Source: CAD feature listing. Evaluate the final solid. Frame: model axes, mm. Face numbers are marked on the shaded views. A direction names the side the tool comes from. Round coordinates to 2 decimals unless told otherwise and drop trailing zeros. Order: outer loops, then holes, each group sorted by start corner. A loop starts at its lowest first (then second) coordinate and runs counter-clockwise, first axis right, second up. Notation, with made-up numbers: (52.5, 23.5) -> (59.5, 23.5) arc R25 cw to (59.5, 43.5) -> close; hole circle Ø7 at (22, -27). An arc over 180 degrees is marked (long way). Use a Markdown table: item, result. Add a question column.
Autodesk Inventor part; units mm, degrees
ref_plane "Arbeitsebene1" through (-25, 25, -22.5) normal (0, 0, 1) x (1, 0, 0)
ref_plane "YZ Plane" through (0, 0, 0) normal (1, 0, 0) x (0, 1, 0)
ref_plane "XZ Plane" through (0, 0, 0) normal (0, 1, 0) x (-1, 0, 0)
sketch "Skizze1" plane through (0, 0, 0) normal (0, 0, 1) x (1, 0, 0)
  line L0 (-25, 25) -> (25, 25)
  line L1 (25, 25) -> (25, -25)
  line L2 (25, -25) -> (-25, -25)
  line L3 (-25, -25) -> (-25, 25)
  line L4 (-35, 0) -> (35, 0)
  line L5 (0, -35) -> (0, 35)
  line L6 (21, 21) -> (-21, 21)
  line L7 (-21, 21) -> (-21, -21)
  line L8 (-21, -21) -> (21, -21)
  line L9 (21, -21) -> (21, 21)
  point P0 (0, 0)
  dimension "d0" = 50
  dimension "d1" = 50
  dimension "d2" = 4
extrude "Extrusion1" add sketch "Skizze1" along normal blind 45 contours L0 L5 L6 L7 L4 L3 | L0 L1 L4 L9 L6 L5 | L4 L7 L8 L5 L2 L3 | L1 L2 L5 L8 L9 L4
sketch "Skizze2" plane through (-25, -25, 0) normal (-1, 0, 0) x (0, 0, 1)
  line L0 (0, 50) -> (45, 50)
  line L1 (0, 0) -> (45, 0)
  line L2 (22.5, 50) -> (22.5, 0)
  line L3 (0, 46) -> (45, 46)
  line L4 (0, 4) -> (45, 4)
  line L5 (0, 46) -> (5, 46)
  line L6 (10, 41) -> (10, 9)
  line L7 (5, 4) -> (0, 4)
  line L8 (0, 4) -> (0, 46)
  line L9 (45, 4) -> (40, 4)
  line L10 (35, 9) -> (35, 41)
  line L11 (40, 46) -> (45, 46)
  line L12 (45, 46) -> (45, 4)
  arc A0 (40, 46) -> (35, 41) centre (40, 41) ccw
  arc A1 (35, 9) -> (40, 4) centre (40, 9) ccw
  arc A2 (5, 4) -> (10, 9) centre (5, 9) ccw
  arc A3 (10, 41) -> (5, 46) centre (5, 41) ccw
  point P0 (0, 25)
  point P1 (10, 4)
  point P2 (35, 46)
  dimension "d5" = 25
  dimension "d6" = 5
extrude "Extrusion2" cut sketch "Skizze2" against normal up to surface (46 mm away) contours A3 L6 A2 L4 L8 L3 | L3 L12 L4 A1 L10 A0
sketch "Skizze4" plane through (-25, -25, 0) normal (0, -1, 0) x (1, 0, 0)
  line L0 (50, 45) -> (0, 45)
  line L1 (0, 0) -> (0, 45)
  line L2 (50, 0) -> (50, 45)
  line L3 (0, 22.5) -> (50, 22.5)
  line L4 (25, 45) -> (25, 0)
  circle A0 centre (25, 22.5) radius 11
  dimension "d19" = 22
extrude "Extrusion3" cut sketch "Skizze4" against normal up to surface (46 mm away) contours A0 L3 L4 | L4 L3 A0 | A0 L4 L3 | L4 A0 L3
mirror "Spiegeln1" about plane through (0, 0, 0) normal (0, 0, 1) of "Extrusion1", "Extrusion2", "Extrusion3"
sketch "Skizze5" plane through (-25, 25, 45) normal (0, 1, 0) x (1, 0, 0)
  circle A0 centre (33.6603, 27.5) radius 3.45
  circle A1 centre (16.3397, 27.5) radius 3.45
  circle A2 centre (25, 12.5) radius 3.45
  line L0 (0, 0) -> (50, 0)
  line L1 (50, 0) -> (50, 90)
  line L2 (60, 45) -> (-10, 45)
  line L3 (50, 45) -> (0, 45)
  line L4 (0, 45) -> (0, 0)
  line L5 (0, 0) -> (50, 0)
  line L6 (50, 0) -> (50, 45)
  point P0 (25, 45)
extrude "Extrusion4" cut sketch "Skizze5" against normal through all contours A0 | A1 | A2 | L4 L2 L1 L0
sketch "Skizze10" plane through (-25, -16, -10) normal (-1, 0, 0) x (0, 0, 1)
  circle A0 centre (-20.5, 16) radius 1.7
  circle A1 centre (-4.5, 16) radius 1.7
  point P0 (10, 16)
hole "Bohrung6" at (-25, 0, -14.5) at (-25, 0, -30.5) direction (1, 0, 0) diameter 2.459 end up to surface
sketch "Skizze11" plane through (-25, -16, -10) normal (-1, 0, 0) x (0, 0, 1)
  line L0 (0, 0) -> (0, 32)
  line L1 (-35, 41) -> (10, 41)
  line L2 (-25, 32) -> (-25, 0)
  line L3 (10, -9) -> (-35, -9)
  line L4 (-12.5, 41) -> (-12.5, -9)
  line L5 (0, 16) -> (-25, 16)
  point P0 (10, 16)
  point P1 (-12.5, 16)
hole "Bohrung7" at (-25, 0, -22.5) direction (1, 0, 0) diameter 5.5 end up to surface
sketch "Skizze12" plane through (-25, -16, -10) normal (-1, 0, 0) x (0, 0, 1)
  line L0 (0, 0) -> (0, 32)
  line L1 (-35, 41) -> (10, 41)
  line L2 (-25, 32) -> (-25, 0)
  line L3 (10, -9) -> (-35, -9)
  line L4 (-12.5, 41) -> (-12.5, -9)
  line L5 (-25, 16) -> (0, 16)
  point P0 (10, 16)
  point P1 (-12.5, 26)
  point P2 (-12.5, 6)
  dimension "d67" = 20
hole "Bohrung8" at (-25, 10, -22.5) at (-25, -10, -22.5) direction (1, 0, 0) diameter 8.5 end up to surface
sketch "Skizze13" plane through (-25, -25, -45) normal (0, -1, 0) x (1, 0, 0)
  circle A0 centre (25, 22.5) radius 11
  line L0 (-10, 45) -> (60, 45)
  line L1 (25, 54) -> (25, -9)
  line L2 (9.5, 38) -> (40.5, 38)
  line L3 (40.5, 38) -> (40.5, 7)
  line L4 (40.5, 7) -> (9.5, 7)
  line L5 (9.5, 7) -> (9.5, 38)
  line L6 (25, 22.5) -> (30.7516, 22.5)
  point P0 (25, 45)
  dimension "d75" = 31
hole "Bohrung9" at (-15.5, -25, -7) at (15.5, -25, -7) at (15.5, -25, -38) at (-15.5, -25, -38) direction (0, 1, 0) diameter 3.4 end through all
sketch "Skizze14" plane through (-25, 25, -45) normal (0, 1, 0) x (1, 0, 0)
  circle A0 centre (9.5, -7) radius 1.7
  circle A1 centre (40.5, -7) radius 1.7
  circle A2 centre (40.5, -38) radius 1.7
  circle A3 centre (9.5, -38) radius 1.7
  point P0 (25, -45)
hole "Bohrung10" at (-15.5, 25, -38) at (15.5, 25, -38) at (15.5, 25, -7) at (-15.5, 25, -7) direction (0, -1, 0) diameter 6 depth 8 tip angle 118
sketch "Skizze15" plane through (-25, 25, 0) normal (0, 0, 1) x (1, 0, 0)
  line L0 (0, -50) -> (0, -46)
  line L1 (50, -50) -> (0, -50)
  line L2 (50, 0) -> (50, -50)
  line L3 (0, 0) -> (50, 0)
  line L4 (2, -2) -> (48, -2)
  line L5 (48, -2) -> (48, -48)
  line L6 (48, -48) -> (2, -48)
  line L7 (2, -48) -> (2, -2)
  point P0 (25, -25)
  dimension "d90" = 2
  dimension "d91" = 2
  dimension "d92" = 2
  dimension "d93" = 2
hole "Bohrung11" at (-23, 23, 0) at (23, 23, 0) at (23, -23, 0) at (-23, -23, 0) direction (0, 0, -1) diameter 1.567 depth 8 tip angle 118
ref_plane "Arbeitsebene1" through (-25, 25, -22.5) normal (0, 0, 1) x (1, 0, 0)
mirror "Spiegeln2" about plane through (-25, 25, -22.5) normal (0, 0, 1) of "Bohrung11"
properties part number "1_0204_002"
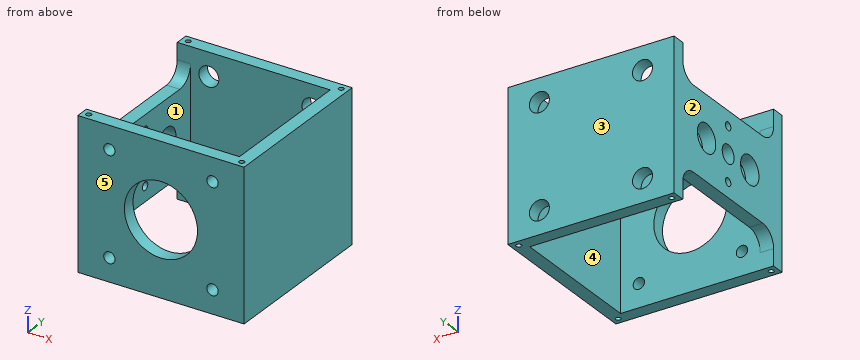
1) Reachability of the marked faces 4 and 5 from +Z, -Z, +X, -X, +Y, -Y: full face, straight path, thin tool, end or side. Return the list, or none.
2) Line query: probe 1 along X at (y, z) = (-23, -5); probe 2 along Z at (x, y) = (-23.75, 0); probe 3 along X at (y, z) = (-14, -17.5). Output: solid intervals per line, ascending. Write a range as from..to.
3) Draft query along Y for the marked faces 1, 2 and 3. Return one class per face: pulls with the +Y half, pulls with the -Y half, needs draft (parallel to the pull), parting line crosses it, or undercut.
4) Section A-A on x = -15.5. Output: boundary loops of the cut face in (y, z), then the cut area to 3 significant figures.
5) Section B-B on y = -19. Output: boundary loops of the cut face in (x, z), then the cut area to 3 significant figures.
6) Section C-C on z = -38. Count the separate pieces of the cut face and the enclosed holes in it, then the cut area to 3 significant figures.
7) Section D-D on x = 0. Output: boundary loops of the cut face in (y, z).
8) First-contact query: pin 1 Ø4.5 at (y, z) = (0, -22.5) entering from -X; pin 2 Ø1.3 at (x, y) = (23, -23) entering from -Z; pin 3 Ø3 at (x, y) = (-24, -4) entering from -Z; pin 4 Ø2 at (x, y) = (19.5, -7) entering from +Z. Flat tips, straight axial feed; report the tip coordinate or a pass-through.
Conclusion:
| question | item | result |
|---|---|---|
| 1 | face 4 | +Z, -Z |
| 1 | face 5 | +Z, -Z, +X, -X, -Y |
| 2 | probe 1 | x = -25..-23.78, -22.22..22.22, 23.78..25 |
| 2 | probe 2 | z = -35..-31.73, -29.27..-25.25, -19.75..-15.73, -13.27..-10 |
| 2 | probe 3 | x = -25..-21, 21..25 |
| 3 | face 1 | undercut |
| 3 | face 2 | needs draft |
| 3 | face 3 | pulls with the +Y half |
| 4 | outline | (-25, -45) -> (-21, -45) -> (-21, -39.7) -> (-25, -39.7) -> close; (-25, -36.3) -> (-21, -36.3) -> (-21, -8.7) -> (-25, -8.7) -> close; (-25, -5.3) -> (-21, -5.3) -> (-21, 0) -> (-25, 0) -> close; (21, -45) -> (25, -45) -> (25, -41) -> (21, -41) -> close; (21, -35) -> (25, -35) -> (25, -10) -> (21, -10) -> close; (21, -4) -> (25, -4) -> (25, 0) -> (21, 0) -> close |
| 4 | area | 285 mm^2 |
| 5 | outline | (-25, -36) -> (-21, -36) -> (-21, -9) -> (-25, -9) -> close; (21, -45) -> (25, -45) -> (25, 0) -> (21, 0) -> close |
| 5 | area | 288 mm^2 |
| 6 | separate pieces | 5 |
| 6 | enclosed holes | 4 |
| 6 | area | 488 mm^2 |
| 7 | outline | (-25, -45) -> (-21, -45) -> (-21, -33.5) -> (-25, -33.5) -> close; (-25, -11.5) -> (-21, -11.5) -> (-21, 0) -> (-25, 0) -> close; (21, -45) -> (25, -45) -> (25, 0) -> (21, 0) -> close |
| 8 | pin 1 | stops at x = 21 |
| 8 | pin 2 | stops at z = -36.92 |
| 8 | pin 3 | stops at z = -35 |
| 8 | pin 4 | passes through |
